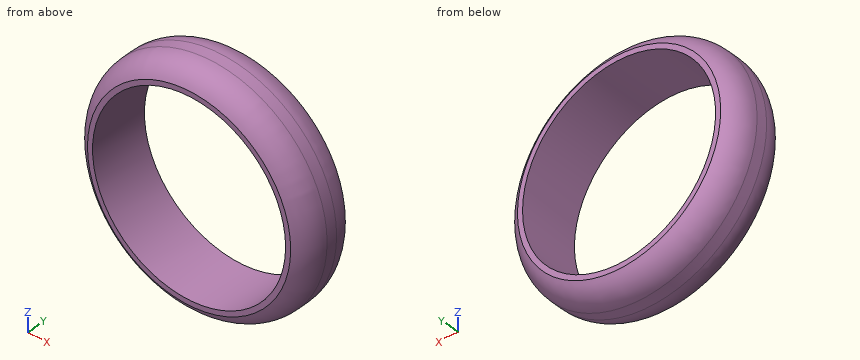
from build123d import *

# Parameters (mm, degrees)
F0_R     = 11.5
F0_R_2   = 10
F1_DEPTH = 6
F0_R_3   = 9.5
F3_DEPTH = 6


# Not quite as in the source:
# - a fillet or chamfer that OpenCascade refuses, or shapes differently, is made with other operations: its cross-section is extruded or revolved along the edge and cut away or added


with BuildPart() as f1:
    # F0 (on Front) → F1 (new body)
    with BuildSketch(Plane.XZ):
        Circle(F0_R)
        Circle(F0_R_2, mode=Mode.SUBTRACT)
    extrude(amount=F1_DEPTH)

    # F2: fillet of radius 2.75 on 3 edges, made by hand

    # F2_s1 → F2_t2 (revolve, cut)
    with BuildSketch(Plane.XY):
        with BuildLine():
            ThreePointArc((11.5, -2.4494897428), (11.0952078799, -1.0133490811), (10, 0))
            Line((10, 0), (11.5, 0))
            Line((11.5, 0), (11.5, -2.4494897428))
        make_face()
    revolve(axis=Axis((0, 0, 0), (0, -1, 0)), mode=Mode.SUBTRACT)

    # F2_s3 → F2_t4 (revolve, cut)
    with BuildSketch(Plane.XY):
        with BuildLine():
            ThreePointArc((11.5, -3.5505102572), (11.0952078799, -4.9866509189), (10, -6))
            Line((10, -6), (11.5, -6))
            Line((11.5, -6), (11.5, -3.5505102572))
        make_face()
    revolve(axis=Axis((0, -6, 0), (0, -1, 0)), mode=Mode.SUBTRACT)

    # F0 (on Front) → F3 (join)
    with BuildSketch(Plane.XZ):
        Circle(F0_R_2)
        Circle(F0_R_3, mode=Mode.SUBTRACT)
    extrude(amount=F3_DEPTH)


solid = f1.part
Read the model definition and answer for the solid it produces. Units are mm, in the model's axes. Round coordinates to 2 decimals unless told otherwise and drop trailing zeros. Write each loop counter-clockwise with the first axis right and the second up, starting at its lowest first coordinate (ties: lowest second). Pieces come first, ordered by that corner, then holes. Notation, with made-up numbers: M 12,47 L 28,47 A26 cw 28,84 Z; hole C 15,10.25 d4. An arc over 180 degrees is marked long. Use a Markdown table: item, result.
1) Flat-ended cylindrical pins translate along their axes: pin 1 (1.5 mm diameter, centred on y = -5, z = -5.5, fed in from -X); pin 2 (3 mm diameter, centred on y = -2, z = -5.5, fed in from -X); pin 3 (1.5 mm diameter, centred on x = 1.5, y = -5, fed in from -Z). Find the tip coordinate at first contact, or state that the pin passes through.
Answers follow:
| item | result |
|---|---|
| pin 1 | stops at x = -10.2 |
| pin 2 | stops at x = -10.77 |
| pin 3 | stops at z = -11.33 |
2) The part is cut by section D-D (y = -4.6). Write down the section's boundary in (x, z).
Answers follow:
| item | result |
|---|---|
| outline | C 0,0 d22.58; hole C 0,0 d19 |
3) The part is cut by section A-A (x = 0). Write down the section's boundary in (y, z).
Answers follow:
| item | result |
|---|---|
| outline | M -6,-10 A2.75 ccw -3.55,-11.5 L -2.45,-11.5 A2.75 ccw 0,-10 L 0,-9.5 L -6,-9.5 Z; M -6,9.5 L 0,9.5 L 0,10 A2.75 ccw -2.45,11.5 L -3.55,11.5 A2.75 ccw -6,10 Z |
4) The part is cut by section C-C (y = -2.1). Write down the section's boundary in (x, z), plus the area to 3 significant figures.
Answers follow:
| item | result |
|---|---|
| outline | C 0,0 d22.96; hole C 0,0 d19 |
| area | 130 mm2 |
5) Straight lines are drawn through the part: line 1 along X through (y, z) = (-3.55, 0.25); line 2 along X through (y, z) = (-2.05, -8.5). For each, find the intervals that lie inside material, in ascending order. Write a range as [from, to].
Answers follow:
| item | result |
|---|---|
| line 1 | x = [-11.5, -9.5], [9.5, 11.5] |
| line 2 | x = [-7.7, -4.24], [4.24, 7.7] |
6) The part is cut by section B-B (z = 0). Write down the section's boundary in (x, y).
Answers follow:
| item | result |
|---|---|
| outline | M -11.5,-3.55 A2.75 ccw -10,-6 L -9.5,-6 L -9.5,0 L -10,0 A2.75 ccw -11.5,-2.45 Z; M 9.5,-6 L 10,-6 A2.75 ccw 11.5,-3.55 L 11.5,-2.45 A2.75 ccw 10,0 L 9.5,0 Z |
